Design review of the part built by this model. Coordinates are the model's own, in mm. A direction names the side the tool comes from. Coordinates: 2 decimals unless noted, no trailing zeros. Order: outer loops, then holes, each group sorted by start corner. A loop starts at its lowest first (then second) coordinate and runs counter-clockwise, first axis right, second up. Notation, with made-up numbers: (52.25, 47) -> (108.25, 47) arc R15 ccw to (108.25, 65) -> close; hole circle Ø6 at (-22.75, 18.5). An arc over 180 degrees is marked (long way). Use a Markdown table: item, result. Add a question column.
Q1. Insertion check: pin 1 (3.5 mm diameter, centred on x = -77.5, z = 80, fed in from +Y); pin 2 (5 mm diameter, centred on y = -6, z = -22.5, fed in from -X). Each pin has a flat end and moves straight along its axis. Give the tip position at first contact, or say it passes through.
Q2. Wall thickness on probe 1 along Z at (x, y) = (-49, -30); probe 2 along X at (y, z) = (0, -65); probe 3 along Y at (x, z) = (2.5, -98.9): over which ranges is each line inside the solid? List them lowest first.
Q3. Add section B-B (x = -18). State the section outline as (y, z) points, then the cut area to 3 significant figures.
Q4. Add section A-A (y = -10). State the section outline as (x, z) points, then the cut area to 3 significant figures.
Q5. The part is to be moulded in two halves that separate along Z. For faces 3 (the face through (1, 1, 1)), 4 (the face through (0, -25, 98)), 5 (the face through (-1, -24, -100)), say which applies: pulls with the +Z half, pulls with the -Z half, needs draft (parallel to the pull), parting line crosses it, or undercut.
Q6. Add section C-C (z = 21). State the section outline as (x, y) points, then the cut area to 3 significant figures.
Q7. Machinability: for faces 1 (the face through (85.5, -25, -1)), 2 (the face through (87.5, -24, -1)), which of the approach directions +Z, -Z, +X, -X, +Y, -Y give a long, thin tool a straight path to every point of the face, cutting with its end or side? Answer none if there is none.
Autodesk Inventor part; units mm, degrees
ref_plane "YZ Plane" through (0, 0, 0) normal (1, 0, 0) x (0, 1, 0)
ref_plane "XZ Plane" through (0, 0, 0) normal (0, 1, 0) x (-1, 0, 0)
ref_plane "XY Plane" through (0, 0, 0) normal (0, 0, 1) x (1, 0, 0)
sketch "Skizze1" plane through (0, 0, 0) normal (0, 1, 0) x (-1, 0, 0)
  line L0 (87.5, -100) -> (-87.5, -100)
  line L1 (-87.5, -100) -> (-87.5, 100)
  line L2 (-87.5, 100) -> (87.5, 100)
  line L3 (87.5, 100) -> (87.5, -100)
  line L4 (0, -140) -> (0, 140)
  line L5 (-122.5, 0) -> (122.5, 0)
  point P0 (0, 0)
  dimension "d0" = 175
  dimension "d1" = 200
extrude "Extrusion1" add sketch "Skizze1" along normal mid plane 2
sketch "Skizze2" plane through (0, -1, 0) normal (0, -1, 0) x (1, 0, 0)
  line L0 (-87.5, -100) -> (-87.5, 100)
  line L1 (87.5, 100) -> (87.5, -100)
  line L2 (-87.5, 100) -> (87.5, 100)
  line L3 (87.5, 100) -> (87.5, 98)
  line L4 (87.5, 98) -> (-87.5, 98)
  line L5 (-87.5, 98) -> (-87.5, 100)
  line L6 (87.5, -100) -> (-87.5, -100)
  line L7 (-87.5, -100) -> (87.5, -100)
  line L8 (87.5, -100) -> (87.5, -98)
  line L9 (87.5, -98) -> (-87.5, -98)
  line L10 (-87.5, -98) -> (-87.5, -100)
  line L11 (87.5, -98) -> (85.5, -98)
  line L12 (85.5, -98) -> (85.5, 98)
  line L13 (85.5, 98) -> (87.5, 98)
  line L14 (87.5, 98) -> (87.5, -98)
  point P0 (0, 0)
  dimension "d4" = 2
  dimension "d5" = 2
  dimension "d6" = 2
extrude "Extrusion2" add sketch "Skizze2" along normal blind 48 contours L0 L9 L1 L6 | L0 L2 L1 L4 | L12 L4 L1 L9
sketch "Skizze3" plane through (0, 1, 0) normal (0, 1, 0) x (1, 0, 0)
  circle A0 centre (-77.5, -80) radius 1.6
  circle A1 centre (-77.5, -65) radius 1.6
  circle A2 centre (-77.5, 80) radius 1.6
  circle A3 centre (-77.5, 65) radius 1.6
  line L0 (-87.5, 100) -> (-87.5, -100)
  line L1 (-87.5, -100) -> (87.5, -100)
  line L2 (87.5, 100) -> (-87.5, 100)
  point P0 (0, 0)
  dimension "d9" = 3.2
  dimension "d10" = 3.2
  dimension "d11" = 3.2
  dimension "d12" = 3.2
  dimension "d13" = 10
  dimension "d14" = 10
  dimension "d15" = 15
  dimension "d16" = 20
  dimension "d17" = 10
  dimension "d18" = 10
  dimension "d19" = 20
  dimension "d20" = 15
extrude "Extrusion3" cut sketch "Skizze3" against normal up to surface (2 mm away)
sketch "Skizze4" plane through (-87.5, 1, 100) normal (0, 0, 1) x (1, 0, 0)
  circle A0 centre (90, -45) radius 1.6
  line L0 (175, -50) -> (175, 0)
  line L1 (175, -50) -> (0, -50)
  point P0 (87.5, -1)
  dimension "d23" = 3.2
  dimension "d24" = 85
  dimension "d25" = 5
extrude "Extrusion4" cut sketch "Skizze4" against normal up to surface (2 mm away)
sketch "Skizze5" plane through (87.5, 1, -100) normal (0, 0, -1) x (-1, 0, 0)
  circle A0 centre (85, -45) radius 1.6
  line L0 (175, -50) -> (0, -50)
  line L1 (0, -50) -> (0, 0)
  point P0 (87.5, -1)
  dimension "d28" = 3.2
  dimension "d29" = 5
  dimension "d30" = 85
extrude "Extrusion5" cut sketch "Skizze5" against normal up to surface (2 mm away)
properties part number "_3D-Druck"
Established:
| question | item | result |
|---|---|---|
| 1 | pin 1 | y = 1 |
| 1 | pin 2 | x = 85.5 |
| 2 | probe 1 | -100 to -98, 98 to 100 |
| 2 | probe 2 | -87.5 to -79.1, -75.9 to 87.5 |
| 2 | probe 3 | -49 to -45.6, -42.4 to 1 |
| 3 | outline | (-49, -100) -> (1, -100) -> (1, 100) -> (-49, 100) -> (-49, 98) -> (-1, 98) -> (-1, -98) -> (-49, -98) -> close |
| 3 | area | 592 mm^2 |
| 4 | outline | (-87.5, -100) -> (87.5, -100) -> (87.5, 100) -> (-87.5, 100) -> (-87.5, 98) -> (85.5, 98) -> (85.5, -98) -> (-87.5, -98) -> close |
| 4 | area | 1,090 mm^2 |
| 5 | face 3 | needs draft |
| 5 | face 4 | undercut |
| 5 | face 5 | pulls with the -Z half |
| 6 | outline | (-87.5, -1) -> (85.5, -1) -> (85.5, -49) -> (87.5, -49) -> (87.5, 1) -> (-87.5, 1) -> close |
| 6 | area | 446 mm^2 |
| 7 | face 1 | -X, -Y |
| 7 | face 2 | +Z, -Z, +X, +Y, -Y |
